Input: part model. Units: mm. Frame: model coordinates. Give positions to 0.01 mm unless a question says otherwise; leave off trailing zeros. Loops run counter-clockwise (first coordinate to the right, second up) from the corner with the lowest first, then second, coordinate; pieces in that order, holes last. Notation, with made-up numbers: M 79,22.5 L 135,22.5 A16 cw 135,29.5 Z; hole C -11.75,74 d1. An arc over 180 degrees is marked long. Use CSV: the item, a comma, the result in double quotes. Start each with the question number.
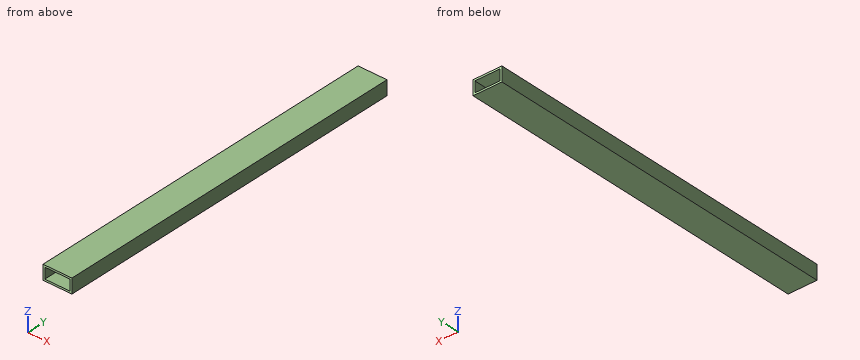
Autodesk Inventor part; units mm, degrees
ref_plane "YZ Plane" through (0, 0, 0) normal (1, 0, 0) x (0, 1, 0)
ref_plane "XZ Plane" through (0, 0, 0) normal (0, 1, 0) x (-1, 0, 0)
ref_plane "XY Plane" through (0, 0, 0) normal (0, 0, 1) x (1, 0, 0)
sketch "Sketch1" plane through (0, 0, 0) normal (0, 1, 0) x (-1, 0, 0)
  line L0 (0, 0) -> (-50.8, 0)
  line L1 (-50.8, 0) -> (-50.8, -25.4)
  line L2 (-50.8, -25.4) -> (0, -25.4)
  line L3 (0, -25.4) -> (0, 0)
  line L4 (-3.175, -22.225) -> (-47.625, -22.225)
  line L5 (-47.625, -22.225) -> (-47.625, -3.175)
  line L6 (-47.625, -3.175) -> (-3.175, -3.175)
  line L7 (-3.175, -3.175) -> (-3.175, -22.225)
  dimension "d0" = 25.4
  dimension "d1" = 50.8
  dimension "d2" = 3.175
  dimension "d3" = 3.175
  dimension "d4" = 3.175
  dimension "d5" = 3.175
extrude "Extrusion1" add sketch "Sketch1" along normal blind 736.6
sketch "Sketch2" plane through (0, 736.6, 0) normal (0, 1, 0) x (1, 0, 0)
  line L0 (-32.6558, 46.2997) -> (107.3615, 46.2997)
  line L1 (107.3615, 46.2997) -> (107.3615, -26.8404)
  line L2 (107.3615, -26.8404) -> (-32.6558, -26.8404)
  line L3 (-32.6558, -26.8404) -> (-32.6558, 46.2997)
  point P0 (0, 0)
extrude "Extrusion2" cut sketch "Sketch2" against normal blind 101.6
properties part number "29in 2x1" material "Aluminum 6061"
Item 1: Section C-C (y = 167). Output: boundary loops of the cut face in (x, z) (3 decimals), then the cut area to 3 significant figures.
Item 2: Section A-A (z = -8.5). Output: boundary loops of the cut face in (x, y) (3 decimals).
Item 3: Section B-B (x = 39.5). Output: boundary loops of the cut face in (y, z) (3 decimals).
Item 4: Material intervals for line 1 (Z direction, x = 30.5, y = 99) (3 decimals); line 2 (X direction, y = 141, z = -4.75) (3 decimals), sorted ascending.
Recorded:
1,outline,"M 0,-25.4 L 50.8,-25.4 L 50.8,0 L 0,0 Z; hole M 3.175,-22.225 L 47.625,-22.225 L 47.625,-3.175 L 3.175,-3.175 Z"
1,area,"444 mm²"
2,outline,"M 0,0 L 3.175,0 L 3.175,635 L 0,635 Z; M 47.625,0 L 50.8,0 L 50.8,635 L 47.625,635 Z"
3,outline,"M 0,-25.4 L 635,-25.4 L 635,-22.225 L 0,-22.225 Z; M 0,-3.175 L 635,-3.175 L 635,0 L 0,0 Z"
4,line 1,"-25.4 to -22.225, -3.175 to 0"
4,line 2,"0 to 3.175, 47.625 to 50.8"
